Design review of the part built by this model. Coordinates are the model's own, in mm. Face numbers are marked on the shaded views. A direction names the side the tool comes from. Coordinates: 2 decimals unless noted, no trailing zeros. Write each loop counter-clockwise with the first axis right and the second up, starting at its lowest first coordinate (ties: lowest second). Pieces come first, ordered by that corner, then holes. Notation, with made-up numbers: (33.5, 1) - (47.5, 1) arc R15 ccw to (47.5, 16) - close; hole circle Ø5 at (26.25, 49). An arc over 180 degrees is marked (long way). One line per item, written item: value.
from build123d import *

# Parameters (mm, degrees)
BOSS_EXTRUDE1_DEPTH = 63
SKETCH2_R           = 16
BOSS_EXTRUDE2_DEPTH = 38
BOSS_EXTRUDE3_DEPTH = 25
CUT_EXTRUDE1_START  = -38
CUT_EXTRUDE1_DEPTH  = 38
CUT_EXTRUDE2_START  = -38
SKETCH2_5_R         = 16
CUT_EXTRUDE2_DEPTH  = 38
BOSS_EXTRUDE4_DEPTH = 65
SKETCH5_R           = 9
CUT_EXTRUDE4_DEPTH  = 38
SKETCH6_R           = 9
CUT_EXTRUDE5_DEPTH  = 38
FILLET1_R           = 25
CUT_EXTRUDE6_DEPTH  = 38


with BuildPart() as part:
    # Sketch1 → Boss-Extrude1 (new, symmetric)
    with BuildSketch(Plane.XY):
        Polygon((0, 0), (0, 90), (13, 90), (13, 13), (78, 13), (78, 0), align=None)
    extrude(amount=BOSS_EXTRUDE1_DEPTH, both=True)

    # Sketch2 → Boss-Extrude2 (add)
    with BuildSketch(Plane(origin=(13, 0, 0), x_dir=(0, 0, -1), z_dir=(1, 0, 0))):
        with BuildLine():
            ThreePointArc((19, 67.248076809), (0, 76), (-19, 67.248076809))
            ThreePointArc((-19, 67.248076809), (-24.031145784, 44.107683096), (-7.5, 27.151519965))
            Line((-7.5, 27.151519965), (7.5, 27.151519965))
            ThreePointArc((7.5, 27.151519965), (20.155644371, 36.209800542), (25, 51))
            ThreePointArc((25, 51), (23.452078799, 59.660254038), (19, 67.248076809))
        make_face()
        with Locations((0, 51)):
            Circle(SKETCH2_R, mode=Mode.SUBTRACT)
    extrude(amount=BOSS_EXTRUDE2_DEPTH)

    # Sketch2<3> → Boss-Extrude3 (add)
    with BuildSketch(Plane(origin=(13, 0, 0), x_dir=(0, 0, -1), z_dir=(1, 0, 0))):
        with BuildLine():
            Line((-9, 90), (-19, 90))
            Line((-19, 90), (-19, 67.248076809))
            ThreePointArc((-19, 67.248076809), (0, 76), (19, 67.248076809))
            Line((19, 67.248076809), (19, 90))
            Line((19, 90), (9, 90))
            ThreePointArc((9, 90), (0, 81), (-9, 90))
        make_face()
    extrude(amount=BOSS_EXTRUDE3_DEPTH)

    # Sketch2<4> → Cut-Extrude1 (cut)
    with BuildSketch(Plane(origin=(13, 0, 0), x_dir=(0, 0, -1), z_dir=(1, 0, 0)).offset(CUT_EXTRUDE1_START)):
        with BuildLine():
            Line((9, 90), (-9, 90))
            ThreePointArc((-9, 90), (0, 81), (9, 90))
        make_face()
    extrude(amount=CUT_EXTRUDE1_DEPTH, mode=Mode.SUBTRACT)

    # Sketch2<5> → Cut-Extrude2 (cut)
    with BuildSketch(Plane(origin=(13, 0, 0), x_dir=(0, 0, -1), z_dir=(1, 0, 0)).offset(CUT_EXTRUDE2_START)):
        with Locations((0, 51)):
            Circle(SKETCH2_5_R)
    extrude(amount=CUT_EXTRUDE2_DEPTH, mode=Mode.SUBTRACT)

    # Sketch2<6> → Boss-Extrude4 (add)
    with BuildSketch(Plane(origin=(13, 0, 0), x_dir=(0, 0, -1), z_dir=(1, 0, 0))):
        with BuildLine():
            ThreePointArc((7.5, 27.151519965), (0, 26), (-7.5, 27.151519965))
            Line((-7.5, 27.151519965), (-7.5, 13))
            Line((-7.5, 13), (7.5, 13))
            Line((7.5, 13), (7.5, 27.151519965))
        make_face()
        with BuildLine():
            Line((7.5, 27.151519965), (-7.5, 27.151519965))
            ThreePointArc((-7.5, 27.151519965), (0, 26), (7.5, 27.151519965))
        make_face()
    extrude(amount=BOSS_EXTRUDE4_DEPTH)

    # Sketch5 → Cut-Extrude4 (cut)
    with BuildSketch(Plane(origin=(13, 0, 0), x_dir=(0, 0, -1), z_dir=(1, 0, 0))):
        with Locations((-44, 65)):
            Circle(SKETCH5_R)
    cut_extrude4 = extrude(amount=-CUT_EXTRUDE4_DEPTH, mode=Mode.SUBTRACT)

    # Mirror1: Cut-Extrude4 across plane
    add(cut_extrude4.mirror(Plane.XY), mode=Mode.SUBTRACT)

    # Sketch6 → Cut-Extrude5 (cut)
    with BuildSketch(Plane(origin=(0, 13, 0), x_dir=(1, 0, 0), z_dir=(0, 1, 0))):
        with Locations(Location((53, -44, 0), (0, 0, 180))):
            Circle(SKETCH6_R)
    cut_extrude5 = extrude(amount=-CUT_EXTRUDE5_DEPTH, mode=Mode.SUBTRACT)

    # Mirror2: Cut-Extrude5 across plane
    add(cut_extrude5.mirror(Plane.XY), mode=Mode.SUBTRACT)

    # Fillet1
    fillet1_edges = [part.edges().sort_by_distance(p)[0] for p in [
        (6.5, 90, 63),
        (6.5, 90, -63),
    ]]
    fillet(fillet1_edges, radius=FILLET1_R)

    # Sketch7 → Cut-Extrude6 (cut)
    with BuildSketch(Plane.XY.offset(7.5)):
        Polygon((51, 27.151519965), (78, 13), (78, 27.151519965), align=None)
    extrude(amount=-CUT_EXTRUDE6_DEPTH, mode=Mode.SUBTRACT)


solid = part.part
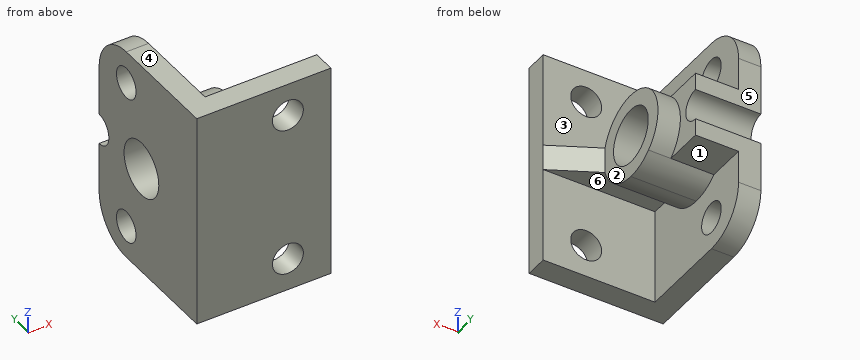
1. Mouldability with a two-part tool opening along Y and no side actions: class the marked faces 4, 5 and 6 as released by +Y, released by -Y, zero draft, split by the parting line, or undercut.
Answer block:
face 4: zero draft
face 5: released by +Y
face 6: undercut
2. Consider section C-C, the plane x = 10.5. Write out the cut boundary in (y, z), then the cut area to 3 significant figures.
Answer block:
outline: (0, -63) - (65, -63) arc R25 ccw to (90, -38) - (90, -9) arc R9 cw to (90, 9) - (90, 38) arc R25 ccw to (65, 63) - (0, 63) - close; hole circle Ø32 at (51, 0); hole circle Ø18 at (65, -44); hole circle Ø18 at (65, 44)
area: 9,630 mm^2
3. Insertion check: pin 1 Ø4 at (x, y) = (37, 16.5) entering from -Z; pin 2 Ø1.5 at (x, z) = (9.5, -1) entering from +Y; pin 3 Ø10 at (x, y) = (51.5, 78.5) entering from -Z. Each pin has a flat end and moves straight along its axis. Give the tip position at first contact, or say it passes through.
Answer block:
pin 1: stops at z = -7.5
pin 2: stops at y = 81.17
pin 3: stops at z = -10.85
4. For the marked faces 1, 2 and 3, list the 3-axis set-ups (+Z, -Z, +X, -X, +Y, -Y) from which the entire face can be reached by the end or side of a thin tool; tool diameter is ignored.
Answer block:
face 1: -Z, +X, +Y
face 2: +Z, -Z, +X, +Y
face 3: +Z, +X
5. Consider section B-B, the plane x = 48.5. Write out the cut boundary in (y, z), then the cut area to 3 significant figures.
Answer block:
outline: (0, -63) - (13, -63) - (13, -51.79) - (0, -51.79) - close; (0, -36.21) - (13, -36.21) - (13, -7.5) - (27.15, -7.5) arc R25 ccw (long way) to (27.15, 7.5) - (13, 7.5) - (13, 36.21) - (0, 36.21) - close; (0, 51.79) - (13, 51.79) - (13, 63) - (0, 63) - close; hole circle Ø32 at (51, 0)
area: 2,590 mm^2
6. Consider section D-D, the plane z = 49. Write out the cut boundary in (x, y).
Answer block:
outline: (0, 0) - (45.52, 0) - (45.52, 13) - (13, 13) - (13, 57.52) - (0, 57.52) - close; (0, 72.48) - (13, 72.48) - (13, 87.45) - (0, 87.45) - close; (60.48, 0) - (78, 0) - (78, 13) - (60.48, 13) - close
7. Consider section A-A, the plane z = 0. Write out the cut boundary in (x, y), then the cut area to 3 significant figures.
Answer block:
outline: (0, 0) - (78, 0) - (78, 13) - (51, 27.15) - (51, 35) - (0, 35) - close; (0, 67) - (51, 67) - (51, 76) - (38, 76) - (38, 81) - (0, 81) - close
area: 2,980 mm^2
8. Wall thickness on line 1 along Z through (x, y) = (53, 4); line 2 along X through (y, z) = (66, -17.5); line 3 along Y through (x, z) = (21, -57): over which ranges is each line inside the solid? List them lowest first.
Answer block:
line 1: z = -63 to -53, -35 to 35, 53 to 63
line 2: x = 0 to 51
line 3: y = 0 to 13
